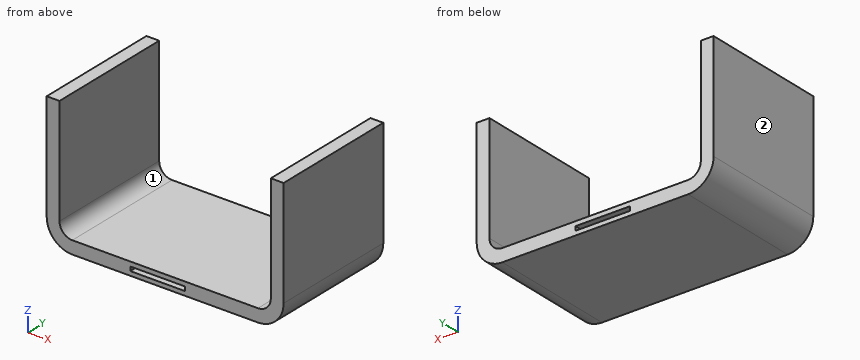
from build123d import *

# Parameters (mm, degrees)
SKETCH1_W           = 8.501053498
SKETCH1_H           = 0.647699314
BOSS_EXTRUDE2_DEPTH = 20


with BuildPart() as part:
    # Sketch1 → Boss-Extrude2 (new body)
    with BuildSketch(Plane(origin=(0, 0, 0), x_dir=(1, 0, 0), z_dir=(0, 1, 0))):
        with BuildLine():
            Line((-16.328355949, -0.789632586), (-16.328355949, 9.010367414))
            Line((-16.328355949, 9.010367414), (-16.328355949, 16.010367414))
            ThreePointArc((-16.328355949, 16.010367414), (-15.742569512, 17.424580976), (-14.328355949, 18.010367414))
            Line((-14.328355949, 18.010367414), (14.671644051, 18.010367414))
            ThreePointArc((14.671644051, 18.010367414), (16.085857613, 17.424580976), (16.671644051, 16.010367414))
            Line((16.671644051, 16.010367414), (16.671644051, 9.010367414))
            Line((16.671644051, 9.010367414), (16.671644051, -0.789632586))
            Line((16.671644051, -0.789632586), (18.671644051, -0.789632586))
            Line((18.671644051, -0.789632586), (18.671644051, 9.010367414))
            Line((18.671644051, 9.010367414), (18.671644051, 16.010367414))
            ThreePointArc((18.671644051, 16.010367414), (17.500071175, 18.838794538), (14.671644051, 20.010367414))
            Line((14.671644051, 20.010367414), (-14.328355949, 20.010367414))
            ThreePointArc((-14.328355949, 20.010367414), (-17.156783074, 18.838794538), (-18.328355949, 16.010367414))
            Line((-18.328355949, 16.010367414), (-18.328355949, 9.010367414))
            Line((-18.328355949, 9.010367414), (-18.328355949, -0.789632586))
            Line((-18.328355949, -0.789632586), (-16.328355949, -0.789632586))
        make_face()
        with Locations((-1.014089745, 19.027186225)):
            Rectangle(SKETCH1_W, SKETCH1_H, mode=Mode.SUBTRACT)
    extrude(amount=BOSS_EXTRUDE2_DEPTH)


solid = part.part
Design review of the part built by this model. Coordinates are the model's own, in mm. Face numbers are marked on the shaded views. A direction names the side the tool comes from. Coordinates: 2 decimals unless noted, no trailing zeros. Order: outer loops, then holes, each group sorted by start corner. A loop starts at its lowest first (then second) coordinate and runs counter-clockwise, first axis right, second up.
Item 1: Take a section at A-A, the plane x = -4.5. Write out the cut boundary in (y, z).
Item 2: Take a section at D-D, the plane x = -12. Write out the cut boundary in (y, z), then the cut area to 3 significant figures.
Item 3: Take a section at C-C, the plane y = 7.5. Write out the cut boundary in (x, z), then the cut area to 3 significant figures.
Item 4: Take a section at B-B, the plane z = -7. Write out the cut boundary in (x, y), then the cut area to 3 significant figures.
Item 5: For line 1 (X direction, y = 5.75, z = -3.25); line 2 (Z direction, x = -2, y = 15.75); line 3 (Z direction, x = 9.5, y = 12.5), list the stretches that pass through material, from the lowest coordinate up.
Item 6: For the marked faces 1 and 2, list the 3-axis set-ups (+Z, -Z, +X, -X, +Y, -Y) from which the entire face can be reached by the end or side of a thin tool; tool diameter is ignored.
Item 7: For pin 1 Ø0.5 at (y, z) = (7, -19) entering from +X; pin 2 Ø2.5 at (x, y) = (-0.5, 8) entering from +Z; pin 3 Ø6 at (x, z) = (-11.5, -14) entering from +Y; pin 4 Ø0.5 at (y, z) = (7.5, -19) entering from -X, all flat-tipped, find the tip position at first contact; note any pin that passes through.
The answers:
1. outline: (0, -20.01) - (20, -20.01) - (20, -19.35) - (0, -19.35) - close; (0, -18.7) - (20, -18.7) - (20, -18.01) - (0, -18.01) - close
2. outline: (0, -20.01) - (20, -20.01) - (20, -18.01) - (0, -18.01) - close
2. area: 40.0 mm2
3. outline: (-18.33, -16.01) arc R4 ccw to (-14.33, -20.01) - (14.67, -20.01) arc R4 ccw to (18.67, -16.01) - (18.67, 0.79) - (16.67, 0.79) - (16.67, -16.01) arc R2 cw to (14.67, -18.01) - (-14.33, -18.01) arc R2 cw to (-16.33, -16.01) - (-16.33, 0.79) - (-18.33, 0.79) - close; hole (-5.26, -19.35) - (3.24, -19.35) - (3.24, -18.7) - (-5.26, -18.7) - close
3. area: 139 mm2
4. outline: (-18.33, 0) - (-16.33, 0) - (-16.33, 20) - (-18.33, 20) - close; (16.67, 0) - (18.67, 0) - (18.67, 20) - (16.67, 20) - close
4. area: 80.0 mm2
5. line 1: x = -18.33 to -16.33, 16.67 to 18.67
5. line 2: z = -20.01 to -19.35, -18.7 to -18.01
5. line 3: z = -20.01 to -18.01
6. face 1: +Z, +Y, -Y
6. face 2: +Z, -Z, -X, +Y, -Y
7. pin 1: stops at x = 17.59
7. pin 2: stops at z = -18.01
7. pin 3: passes through
7. pin 4: stops at x = -17.24
